Verification items for the finished model (mm, model axes). A direction names the side the tool comes from. Coordinates: 2 decimals unless noted, no trailing zeros. Write each loop counter-clockwise with the first axis right and the second up, starting at its lowest first coordinate (ties: lowest second). Pieces come first, ordered by that corner, then holes. Notation, with made-up numbers: (25.25, -16.5) -> (70.25, -16.5) arc R23 cw to (70.25, 0.5) -> close; hole circle Ø4 at (46, 32.25). An arc over 180 degrees is marked (long way). Answer in a Markdown table with one row per item.
```python
from build123d import *

# Parameters (mm, degrees)
SKETCH1_R                = 45
SKETCH1_R_2              = 42.5
BOSS_EXTRUDE1_DEPTH      = 10
SKETCH4_R                = 2.5
BOSS_EXTRUDE2_DEPTH      = 5
FILLET1_R                = 3
CIRPATTERN1_COUNT        = 4
FILLET1_OF_CIRPATTERN1_R = 3


with BuildPart() as part:
    # Sketch1 → Boss-Extrude1 (new body)
    with BuildSketch(Plane.XY):
        Circle(SKETCH1_R)
        Circle(SKETCH1_R_2, mode=Mode.SUBTRACT)
    extrude(amount=BOSS_EXTRUDE1_DEPTH)

    # Sketch3 → Revolve1 (revolve)
    with BuildSketch(Plane(origin=(0, 0, 0), x_dir=(0, 0, -1), z_dir=(1, 0, 0))):
        with BuildLine():
            Line((-55, 0), (-52.5, 0))
            ThreePointArc((-52.5, 0), (-40.0520382, -30.0520382), (-10, -42.5))
            Line((-10, -42.5), (-10, -45))
            ThreePointArc((-10, -45), (-41.819805153, -31.819805153), (-55, 0))
        make_face()
    revolve(axis=Axis((0, 0, 55), (0, 0, -1)))

    # Sketch4 → Boss-Extrude2 (add)
    with BuildSketch(Plane.XY):
        with BuildLine():
            Line((5, 44.72135955), (5, 50))
            ThreePointArc((5, 50), (0, 55), (-5, 50))
            Line((-5, 50), (-5, 44.72135955))
            ThreePointArc((-5, 44.72135955), (0, 45), (5, 44.72135955))
        make_face()
        with Locations((0, 50)):
            Circle(SKETCH4_R, mode=Mode.SUBTRACT)
    boss_extrude2 = extrude(amount=BOSS_EXTRUDE2_DEPTH)

    # Fillet1
    fillet1_edges = [part.edges().sort_by_distance(p)[0] for p in [
        (-5, 44.72135955, 2.5),
        (5, 44.72135955, 2.5),
    ]]
    fillet(fillet1_edges, radius=FILLET1_R)

    # CirPattern1: Boss-Extrude2 ×4 about axis
    cirpattern1_axis = Axis((0, 0, 0), (0, 0, 1))
    for i in range(1, CIRPATTERN1_COUNT):
        add(boss_extrude2.rotate(cirpattern1_axis, i * 360 / CIRPATTERN1_COUNT))

    # Fillet1 of CirPattern1
    fillet1_of_cirpattern1_edges = [part.edges().sort_by_distance(p)[0] for p in [
        (-44.72135955, -5, 2.5),
        (-44.72135955, 5, 2.5),
        (5, -44.72135955, 2.5),
        (-5, -44.72135955, 2.5),
        (44.72135955, 5, 2.5),
        (44.72135955, -5, 2.5),
    ]]
    fillet(fillet1_of_cirpattern1_edges, radius=FILLET1_OF_CIRPATTERN1_R)


solid = part.part
```
1. Section check A-A, the plane y = 0. Record the boundary of the cut face in (x, z).
Geometry says:
| item | result |
|---|---|
| outline | (-55, 0) -> (-52.5, 0) -> (-52.5, 5) -> (-55, 5) -> close; (-47.5, 0) -> (-42.5, 0) -> (-42.5, 10) arc R42.5 cw to (42.5, 10) -> (42.5, 0) -> (47.5, 0) -> (47.5, 5) -> (45, 5) -> (45, 10) arc R45 ccw to (-45, 10) -> (-45, 5) -> (-47.5, 5) -> close; (52.5, 0) -> (55, 0) -> (55, 5) -> (52.5, 5) -> close |
2. Mould release check, pull along Y, two halves, no side actions. Record for faces 4 (the flat face through (5, 49, 2)), 5 (the cylindrical face through (-0.54, 47.56, 2.46)), 6 (the cylindrical face through (47.56, 0.54, 2.46)), 7 (the cylindrical face through (5.7, -45.4, 2.5)): released by +Y, released by -Y, zero draft, split by the parting line, or undercut.
Geometry says:
| item | result |
|---|---|
| face 4 | zero draft |
| face 5 | undercut |
| face 6 | undercut |
| face 7 | released by -Y |
3. Tool access check on faces 1 (the flat face through (-5, -49, 2)), 2 (the flat face through (5, -49, 2)), 3 (the flat face through (-49, 5, 2)). Record the directions out of +Z, -Z, +X, -X, +Y, -Y that give a thin tool (end or side, any length) a straight path to the whole face; none if there is none.
Geometry says:
| item | result |
|---|---|
| face 1 | +Z, -Z, -X, -Y |
| face 2 | +Z, -Z, +X, -Y |
| face 3 | +Z, -Z, -X, +Y |
4. Depth check by flat-ended pin: P1, Ø4, axis at x = 34.5, y = 22.5, coming from the -Z side; P2, Ø1.3, axis at y = 48.5, z = 3.5, coming from the -X side; P3, Ø6, axis at x = 50, y = 0, coming from the +Z side; P4, Ø3, axis at y = 49, z = 3, coming from the +X side. Enter the tip coordinate at first touch or a pass-through.
Geometry says:
| item | result |
|---|---|
| P1 | z = 0 |
| P2 | x = -5 |
| P3 | z = 5 |
| P4 | x = 5 |
5. Section check D-D, the plane z = 15. Record the boundary of the cut face in (x, y).
Geometry says:
| item | result |
|---|---|
| outline | circle Ø89.44 at (0, 0); hole circle Ø84.41 at (0, 0) |
6. Thickness scan on line 1 (X direction, y = 0, z = 1.3); line 2 (X direction, y = -50, z = 3.35). Record the ranges inside material, lowest first. Write a range as from..to.
Geometry says:
| item | result |
|---|---|
| line 1 | -55..-52.5, -47.5..-42.5, 42.5..47.5, 52.5..55 |
| line 2 | -5..-2.5, 2.5..5 |
7. Section check C-C, the plane y = -23. Record the boundary of the cut face in (x, z).
Geometry says:
| item | result |
|---|---|
| outline | (-38.68, 0) -> (-35.74, 0) -> (-35.74, 10) arc R35.74 cw to (35.74, 10) -> (35.74, 0) -> (38.68, 0) -> (38.68, 10) arc R38.68 ccw to (-38.68, 10) -> close |
